from build123d import *

# Parameters (mm, degrees)
F0_W     = 37
F0_H     = 10
F0_W_2   = 6
F0_R     = 10
F1_DEPTH = 67.5
F2_W     = 10
F2_H     = 27.5
F3_DEPTH = 250


with BuildPart() as f1:
    # F0 (on Top) → F1 (new body)
    with BuildSketch(Plane.XY):
        Polygon((45, 27.5), (45, 37.5), (-45, 37.5), (-45, 27.5), (-8, 27.5), (-2, 27.5), align=None)
        with Locations((-26.5, 22.5)):
            Rectangle(F0_W, F0_H)
        with Locations((-5, 22.5)):
            Rectangle(F0_W_2, F0_H)
        Polygon((45, 17.5), (45, 27.5), (-2, 27.5), (-2, 17.5), (5, 17.5), align=None)
        with BuildLine():
            Line((45, -17.5), (45, 17.5))
            Line((45, 17.5), (5, 17.5))
            Line((5, 17.5), (5, -17.5))
            ThreePointArc((5, -17.5), (25, 2.5), (45, -17.5))
        make_face()
        with BuildLine():
            Line((-8, 17.5), (-45, 17.5))
            Line((-45, 17.5), (11.781288, -32.508853))
            ThreePointArc((11.781288, -32.508853), (6.773999, -25.734858), (5, -17.5))
            Line((5, -17.5), (5, 17.5))
            Line((5, 17.5), (-2, 17.5))
            Line((-2, 17.5), (-8, 17.5))
        make_face()
        with BuildLine():
            ThreePointArc((11.781288, -32.508853), (33.234858, -35.726001), (45, -17.5))
            ThreePointArc((45, -17.5), (25, 2.5), (5, -17.5))
            ThreePointArc((5, -17.5), (6.773999, -25.734858), (11.781288, -32.508853))
        make_face()
        with Locations((25, -17.5)):
            Circle(F0_R, mode=Mode.SUBTRACT)
    extrude(amount=F1_DEPTH)

    # F2 (on face) → F3 (cut)
    with BuildSketch(Plane(origin=(-45, 0, 0), x_dir=(0, -1, 0), z_dir=(-1, 0, 0))):
        with Locations((-32.5, 13.75)):
            Rectangle(F2_W, F2_H)
    extrude(amount=-F3_DEPTH, mode=Mode.SUBTRACT)


solid = f1.part
The model under review builds one solid part; all positions refer to its coordinate system, in mm. A direction names the side the tool comes from. Round coordinates to 2 decimals unless told otherwise and drop trailing zeros. Write each loop counter-clockwise with the first axis right and the second up, starting at its lowest first coordinate (ties: lowest second). Pieces come first, ordered by that corner, then holes. Notation, with made-up numbers: M 14,-12.5 L 60,-12.5 A32 cw 60,22.5 Z; hole C 50.5,31.5 d6. An arc over 180 degrees is marked long. Use a Markdown table: item, result. Add a question column.
Q1. The part is to be moulded in two halves that separate along Y. For faces 3 (the face through (-1, 27.5, 14)), 4 (the face through (-17.01, -7.15, 33.28)), 5 (the face through (34.54, -14.5, 33.28)), 6 (the face through (9, 9, 67.5)), say which applies: pulls with the +Y half, pulls with the -Y half, needs draft (parallel to the pull), parting line crosses it, or undercut.
Q2. We need section D-D, the plane z = 60. State the section outline as (x, y) points.
Q3. Insertion check: pin 1 (5 mm diameter, centred on x = -29.5, z = 26.5, fed in from -Y); pin 2 (3 mm diameter, centred on x = 13, y = 30.5, fed in from -Z); pin 3 (6 mm diameter, centred on y = -18, z = 47, fed in from -X); pin 4 (5 mm diameter, centred on x = 13.5, y = 22.5, fed in from -Z). Each pin has a flat end and moves straight along its axis. Give the tip position at first contact, or say it passes through.
Q4. We need section B-B, the plane z = 9.5. State the section outline as (x, y) points, plus the area to 3 significant figures.
Q5. We need section A-A, the plane x = 25. State the section outline as (y, z) points.
Q6. We need section C-C, the plane y = -22. State the section outline as (x, z) points.
Q7. Machinability: for faces 1 (the face through (32.941, -35.856, 33.277)), 2 (the face through (-1, 33, 27.5)), which of the approach directions +Z, -Z, +X, -X, +Y, -Y give a long, thin tool a straight path to every point of the face, cutting with its end or side? Answer none if there is none.
Q8. To check wall thickness, follow line 1 (Y direction, x = 25, z = 43); line 2 (X direction, y = -17, z = 31); line 3 (X direction, y = 6.5, z = 61). State the ranges of each line that lie inside material, in increasing order.
Findings below:
| question | item | result |
|---|---|---|
| 1 | face 3 | pulls with the +Y half |
| 1 | face 4 | pulls with the -Y half |
| 1 | face 5 | undercut |
| 1 | face 6 | needs draft |
| 2 | outline | M -45,17.5 L 11.78,-32.51 A20 ccw 45,-17.5 L 45,37.5 L -45,37.5 Z; hole C 25,-17.5 d20 |
| 3 | pin 1 | stops at y = 1.65 |
| 3 | pin 2 | stops at z = 27.5 |
| 3 | pin 3 | stops at x = -8.1 |
| 3 | pin 4 | stops at z = 0 |
| 4 | outline | M -45,17.5 L 11.78,-32.51 A20 ccw 45,-17.5 L 45,27.5 L -45,27.5 Z; hole C 25,-17.5 d20 |
| 4 | area | 3,730 mm² |
| 5 | outline | M -37.5,0 L -27.5,0 L -27.5,67.5 L -37.5,67.5 Z; M -7.5,0 L 27.5,0 L 27.5,27.5 L 37.5,27.5 L 37.5,67.5 L -7.5,67.5 Z |
| 6 | outline | M -0.15,0 L 16.07,0 L 16.07,67.5 L -0.15,67.5 Z; M 33.93,0 L 44.49,0 L 44.49,67.5 L 33.93,67.5 Z |
| 7 | face 1 | +Z, -Z, -Y |
| 7 | face 2 | -Z, +X, -X, +Y |
| 8 | line 1 | y = -37.5 to -27.5, -7.5 to 37.5 |
| 8 | line 2 | x = -5.83 to 15.01, 34.99 to 45 |
| 8 | line 3 | x = -32.51 to 45 |
